Verification items for the finished model (mm, model axes). Round coordinates to 2 decimals unless told otherwise and drop trailing zeros. Write each loop counter-clockwise with the first axis right and the second up, starting at its lowest first coordinate (ties: lowest second). Pieces come first, ordered by that corner, then holes. Notation, with made-up numbers: (49.5, 27) - (77.5, 27) arc R34 cw to (77.5, 57) - close; hole circle Ø1 at (-11.75, 53.25). An arc over 180 degrees is marked (long way). Answer as a JSON object with one key per item and string values.
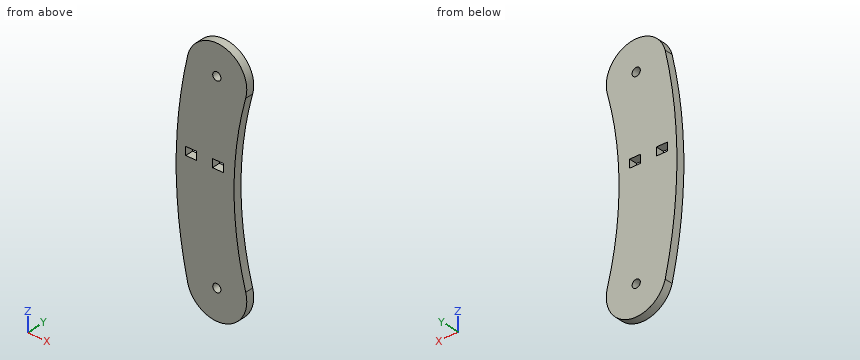
Autodesk Inventor part; units mm, degrees
ref_plane "YZ Plane" through (0, 0, 0) normal (1, 0, 0) x (0, 1, 0)
ref_plane "XZ Plane" through (0, 0, 0) normal (0, 1, 0) x (-1, 0, 0)
ref_plane "XY Plane" through (0, 0, 0) normal (0, 0, 1) x (1, 0, 0)
sketch "Sketch1" plane through (0, 0, 0) normal (0, 1, 0) x (-1, 0, 0)
  arc A0 (13.7652, 13.7563) -> (-7.6488, 8.7996) centre (2.9529, 11.7331) ccw
  arc A1 (-7.6488, -55.3335) -> (13.7652, -60.2902) centre (2.9529, -58.2669) ccw
  arc A2 (-7.6723, -55.4199) -> (-7.6723, 8.8861) centre (-125.5725, -23.2669) ccw
  arc A3 (13.578, -61.1139) -> (13.578, 14.5801) centre (-151.1069, -23.2669) ccw
  circle A4 centre (2.9529, 11.7331) radius 1.5
  circle A5 centre (2.9529, -58.2669) radius 1.5
  line L0 (14.3609, -16.1047) -> (10.3609, -16.1047)
  line L1 (10.3609, -16.1047) -> (10.3609, -19.1047)
  line L2 (10.3609, -19.1047) -> (14.3609, -19.1047)
  line L3 (14.3609, -19.1047) -> (14.3609, -16.1047)
  line L4 (14.3609, -11.7669) -> (10.3609, -14.7669) construction
  line L5 (10.3609, -11.7669) -> (14.3609, -14.7669) construction
  line L6 (0.5448, -16.1047) -> (4.5448, -16.1047)
  line L7 (4.5448, -16.1047) -> (4.5448, -19.1047)
  line L8 (4.5448, -19.1047) -> (0.5448, -19.1047)
  line L9 (0.5448, -19.1047) -> (0.5448, -16.1047)
  line L10 (12.3609, -13.2669) -> (12.3609, -13.2669)
  line L11 (2.9529, 11.7331) -> (2.9529, -58.2669)
  line L12 (10.3609, -18.6047) -> (4.5448, -18.6047)
  line L13 (7.4529, -18.6047) -> (7.4529, -17.6047)
  point P0 (0, 0)
  dimension "d0" = 22
  dimension "d1" = 22
  dimension "d2" = 70
  dimension "d3" = 3
  dimension "d4" = 3
  dimension "d21" = 4
  dimension "d22" = 3
  dimension "d25" = 0
  dimension "d26" = 1
sketch "Sketch2" plane through (0, 0, 0) normal (0, 1, 0) x (-1, 0, 0)
  point P0 (0, 0)
extrude "Extrusion1" add sketch "Sketch1" along normal blind 3 contours A3 A1 A2 A0
sketch "Sketch3" plane through (0, 0, 0) normal (0, -1, 0) x (1, 0, 0)
  point P0 (0, 0)
sketch "Sketch4" plane through (0, 0, 0) normal (0, -1, 0) x (1, 0, 0)
  point P0 (0, 0)
sketch "Sketch5" plane through (0, 3, 0) normal (0, 1, 0) x (1, 0, 0)
  point P0 (0, 0)
sketch "Sketch6" plane through (0, 3, 0) normal (0, 1, 0) x (1, 0, 0)
  point P0 (0, 0)
properties part number "fem2"
1. Cross-section at A-A (x = -12.75). Record the boundary of the cut face in (y, z).
Completed:
{"outline": "(0, -63.27) - (3, -63.27) - (3, -19.1) - (0, -19.1) - close; (0, -16.1) - (3, -16.1) - (3, 16.73) - (0, 16.73) - close"}
2. Cross-section at B-B (y = 1.8). Record the boundary of the cut face in (x, z), plus the area to 3 significant figures.
Completed:
{"outline": "(-13.58, -61.11) arc R11 ccw (long way) to (7.65, -55.33) arc R122.21 cw to (7.65, 8.8) arc R11 ccw (long way) to (-13.58, 14.58) arc R168.98 ccw to start; hole (-14.36, -19.1) - (-10.36, -19.1) - (-10.36, -16.1) - (-14.36, -16.1) - close; hole (-4.54, -19.1) - (-0.54, -19.1) - (-0.54, -16.1) - (-4.54, -16.1) - close; hole circle Ø3 at (-2.95, -58.27); hole circle Ø3 at (-2.95, 11.73)", "area": "1,860 mm^2"}
3. Go/stop test with flat-tipped pins: pin 1 (0.9 mm diameter, centred on y = 1.5, z = -17, fed in from -X); pin 2 (3.5 mm diameter, centred on x = -2.95, z = 11.73, fed in from +Y); pin 3 (1.5 mm diameter, centred on x = -13, y = 2, fed in from -Z); pin 4 (0.9 mm diameter, centred on x = -11.5, y = 2, fed in from +Z). Record where each tip stops, or that it passes through.
Completed:
{"pin 1": "stops at x = -17.77", "pin 2": "stops at y = 3", "pin 3": "stops at z = -64.15", "pin 4": "stops at z = 19.18"}
4. Cross-section at D-D (x = 4.25). Record the boundary of the cut face in (y, z), plus the area to 3 significant figures.
Completed:
{"outline": "(0, -66.58) - (3, -66.58) - (3, -37.93) - (0, -37.93) - close; (0, -8.6) - (3, -8.6) - (3, 20.05) - (0, 20.05) - close", "area": "172 mm^2"}
5. Material ranges on probe 1 along Z at (x, y) = (-2.75, 1.35); probe 2 along Z at (x, y) = (-4, 0.5); probe 3 along X at (y, z) = (2.7, -23.5), recorded low to high. Write a range as from..to.
Completed:
{"probe 1": "z = -69.27..-59.75, -56.78..-19.1, -16.1..10.25, 13.22..22.73", "probe 2": "z = -69.22..-59.34, -57.19..-19.1, -16.1..10.66, 12.81..22.68", "probe 3": "x = -17.87..3.37"}
6. Cross-section at C-C (x = -2.25). Record the boundary of the cut face in (y, z).
Completed:
{"outline": "(0, -69.24) - (3, -69.24) - (3, -59.59) - (0, -59.59) - close; (0, -56.94) - (3, -56.94) - (3, -19.1) - (0, -19.1) - close; (0, -16.1) - (3, -16.1) - (3, 10.41) - (0, 10.41) - close; (0, 13.06) - (3, 13.06) - (3, 22.71) - (0, 22.71) - close"}
